from build123d import *

# Parameters (mm, degrees)
SKETCH2_R           = 11.1125
BOSS_EXTRUDE1_DEPTH = 3.048
SKETCH3_R           = 10.16
CUT_EXTRUDE1_DEPTH  = 1.27
SKETCH4_R           = 3.81
CUT_EXTRUDE2_DEPTH  = 2.54
FILLET1_R           = 10.16


with BuildPart() as part:
    # Sketch2 → Boss-Extrude1 (new body)
    with BuildSketch(Plane(origin=(0, 0, 0), x_dir=(1, 0, 0), z_dir=(0, 1, 0))):
        with Locations(Location((0, 0, 0), (0, 0, 90))):
            Circle(SKETCH2_R)
    extrude(amount=BOSS_EXTRUDE1_DEPTH)

    # Sketch3 → Cut-Extrude1 (cut)
    with BuildSketch(Plane(origin=(0, 3.048, 0), x_dir=(1, 0, 0), z_dir=(0, 1, 0))):
        with Locations(Location((0, 0, 0), (0, 0, 270))):
            Circle(SKETCH3_R)
    extrude(amount=-CUT_EXTRUDE1_DEPTH, mode=Mode.SUBTRACT)

    # Sketch4 → Cut-Extrude2 (cut)
    with BuildSketch(Plane(origin=(0, 0, 0), x_dir=(-1, 0, 0), z_dir=(0, -1, 0))):
        with Locations(Location((0, 0, 0), (0, 0, 90))):
            Circle(SKETCH4_R)
    extrude(amount=-CUT_EXTRUDE2_DEPTH, mode=Mode.SUBTRACT)

    # Fillet1
    # the kernel refuses this fillet: 10.16 mm, written as the material it takes off along each edge
    with BuildSketch(Plane(origin=(0, 0, 0), x_dir=(0, 0, -1), z_dir=(-1, 0, 0))) as fillet1_piece_1:
        with BuildLine():
            CenterArc((9.551748514, -10.16), FILLET1_R, 90, 34.41150867)
            Line((3.81, -1.778), (3.81, 0))
            Line((3.81, 0), (9.551748514, 0))
        make_face()
    revolve(axis=Axis((0, 0, 0), (0, -1, 0)), mode=Mode.SUBTRACT)


solid = part.part
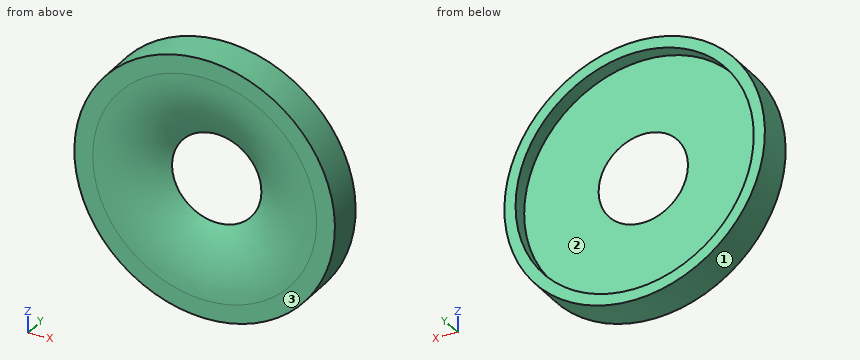
Work out the finished part from the listing and answer in its coordinate system (mm). Face numbers are marked on the shaded views. Give positions to 0.01 mm unless a question says otherwise; leave off trailing zeros. Write each loop counter-clockwise with the first axis right and the second up, starting at its lowest first coordinate (ties: lowest second). Pieces come first, ordered by that corner, then holes. Notation, with made-up numbers: (-6.75, 7.5) - (25.25, 7.5) arc R25 ccw to (25.25, 31.5) - close; hole circle Ø10 at (85, 27.5). An arc over 180 degrees is marked (long way). One line per item, written item: value. Start each with the question number.
1. Consider probe 1 along X at (y, z) = (2.85, 0); probe 2 along Y at (x, z) = (-6.75, 6.25); probe 3 along X at (y, z) = (2.3, -4.5). Determine where each line is inside the solid, lowest interval first.
2. Find section A-A (y = 2.05). Write down the section's boundary in (x, z) (1 decimal), then the cut area to 3 significant figures.
3. Given pin 1 (1 mm diameter, centred on x = 8, z = -9, fed in from +Y); pin 2 (1 mm diameter, centred on x = -6.5, y = 1.5, fed in from +Z); pin 3 (1.5 mm diameter, centred on x = 3.5, y = 1.5, fed in from -Z); pin 4 (1.5 mm diameter, centred on y = 1, z = -2.5, fed in from +X), each flat-ended and moving along its own axis, determine where each tip first touches the part or whether it passes through.
4. For a pull along X with two mould halves and no side action, classify the marked faces 1, 2 and 3 as +X half, -X half, draft (parallel to the pull), parting line (faces both ways), or undercut.
Geometry results:
1. probe 1: -11.11 to -10.16, 10.16 to 11.11
1. probe 2: 0.01 to 1.78
1. probe 3: -10.16 to -9.11, 9.11 to 10.16
2. outline: circle Ø22.2 at (0, 0); hole circle Ø20.3 at (0, 0)
2. area: 63.7 mm2
3. pin 1: through
3. pin 2: z = 9.35
3. pin 3: z = -10.77
3. pin 4: x = 10.97
4. face 1: parting line
4. face 2: undercut
4. face 3: draft
